```python
from build123d import *

# Parameters (mm, degrees)
ESQUISSE1_R                                        = 4
BOSS_EXTRU_1_DEPTH                                 = 8
CHAMBRAGE_POUR_VIS_T_TE_HEXAGONALE_M31_D           = 3.4
CHAMBRAGE_POUR_VIS_T_TE_HEXAGONALE_M31_CBORE_D     = 6.5
CHAMBRAGE_POUR_VIS_T_TE_HEXAGONALE_M31_CBORE_DEPTH = 3.5
CHANFREIN1_SIZE                                    = 0.2


with BuildPart() as part:
    # Esquisse1 → Boss.-Extru.1 (new body)
    with BuildSketch(Plane.XY):
        Circle(ESQUISSE1_R)
    extrude(amount=BOSS_EXTRU_1_DEPTH)

    # Chambrage pour vis à tête hexagonale M31 (through all)
    with Locations(Plane.XY.offset(8)):
        with Locations((0, 0)):
            CounterBoreHole(CHAMBRAGE_POUR_VIS_T_TE_HEXAGONALE_M31_D / 2, CHAMBRAGE_POUR_VIS_T_TE_HEXAGONALE_M31_CBORE_D / 2, CHAMBRAGE_POUR_VIS_T_TE_HEXAGONALE_M31_CBORE_DEPTH)

    # Chanfrein1
    chanfrein1_edges = [part.edges().sort_by_distance(p)[0] for p in [
        (-4, 0, 8),
    ]]
    chamfer(chanfrein1_edges, length=CHANFREIN1_SIZE)


solid = part.part
```
Verification items for the finished model (mm, model axes). A direction names the side the tool comes from. Coordinates: 2 decimals unless noted, no trailing zeros. Loops run counter-clockwise (first coordinate to the right, second up) from the corner with the lowest first, then second, coordinate; pieces in that order, holes last. Notation, with made-up numbers: (53, -28.75) -> (109, -28.75) arc R14 ccw to (109, -13.75) -> close; hole circle Ø6 at (-15, 75). An arc over 180 degrees is marked (long way). Answer in a Markdown table with one row per item. Add a question column.
1. Depth check by flat-ended pin: P1, Ø4, axis at x = 0, y = 0, coming from the +Z side. Enter the tip coordinate at first touch or a pass-through.
2. Section check A-A, the plane x = 0. Enter the section's corners in (y, z).
3. Section check C-C, the plane z = 5.5. Enter the section's corners in (x, y).
4. Access from +Z, -Z, +X, -X, +Y, -Y to the whole of each face (thin tool, end or side, straight path). Record for faces 1 (the face through (-2.579, -1.978, 6.274)), 2 (the face through (2, 0, 0)).
5. Section check D-D, the plane z = 2.25. Enter the section's corners in (x, y).
6. Material ranges on probe 1 along Y at (x, z) = (0, 5.2); probe 2 along Y at (x, z) = (0, 2.4); probe 3 along Z at (x, y) = (-1, 3), recorded low to high. Write a range as [from, to].
7. Draft check along X on faces 3 (the face through (-0.867, -3.905, 3.845)), 4 (the face through (3, 2, 8)), 5 (the face through (1.4, -1.4, 4.5)). Enter one of: +X half, -X half, draft (parallel to the pull), parting line (faces both ways), or undercut.
Derived:
| question | item | result |
|---|---|---|
| 1 | P1 | stops at z = 4.5 |
| 2 | outline | (-4, 0) -> (-1.7, 0) -> (-1.7, 4.5) -> (-3.25, 4.5) -> (-3.25, 8) -> (-3.8, 8) -> (-4, 7.8) -> close; (1.7, 0) -> (4, 0) -> (4, 7.8) -> (3.8, 8) -> (3.25, 8) -> (3.25, 4.5) -> (1.7, 4.5) -> close |
| 3 | outline | circle Ø8 at (0, 0); hole circle Ø6.5 at (0, 0) |
| 4 | face 1 | +Z |
| 4 | face 2 | -Z, +X, -X, +Y, -Y |
| 5 | outline | circle Ø8 at (0, 0); hole circle Ø3.4 at (0, 0) |
| 6 | probe 1 | y = [-4, -3.25], [3.25, 4] |
| 6 | probe 2 | y = [-4, -1.7], [1.7, 4] |
| 6 | probe 3 | z = [0, 4.5] |
| 7 | face 3 | parting line |
| 7 | face 4 | draft |
| 7 | face 5 | undercut |
